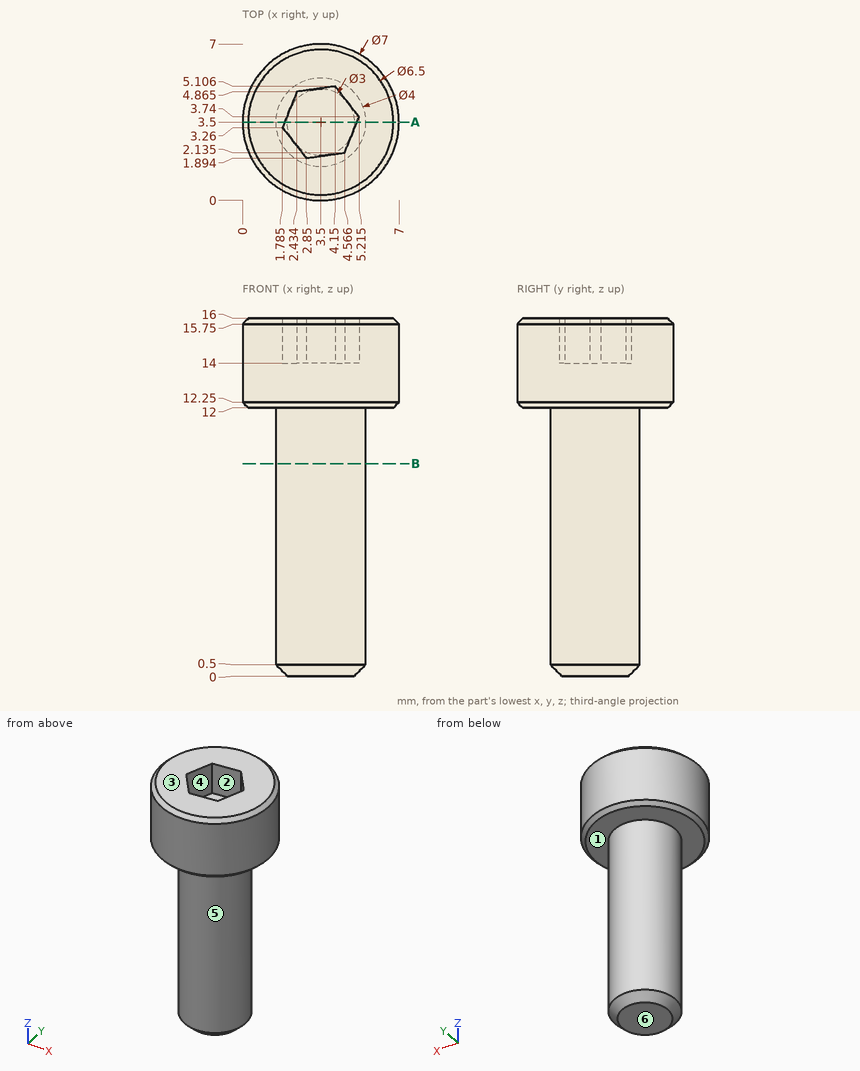
Can you work these out from the drawing? Everything is in mm from the part's minimum corner. A direction names the side the tool comes from. Round coordinates to 2 decimals unless told otherwise and drop trailing zeros. Order: outer loops, then holes, each group sorted by start corner. A loop starts at its lowest first (then second) coordinate and runs counter-clockwise, first axis right, second up. Notation, with made-up numbers: (-18, 50) -> (17, 50) arc R12 ccw to (17, 70) -> close; hole circle Ø4 at (6.25, 76). An arc over 180 degrees is marked (long way). Return JSON: item names as keys, results as strings. Group by question number.
1. If we section it at A-A, the plane y = 3.5: Write out the boundary of the cut face in (x, z).
2. I need wall thicknesses on line 1 (Z direction, x = 4, y = 3.75); line 2 (Z direction, x = 2, y = 6); line 3 (X direction, y = 4.25, z = 9.25) (1 decimal). Which ranges of each line are inside material? Lowest first, please. Write a range as [from, to].
3. If we section it at B-B, the plane z = 9.5: Write out the boundary of the cut face in (x, y).
4. We'd pull the mould along X, two halves only. Please class the marked faces 4, 5 and 6: released by +X, released by -X, zero draft, split by the parting line, or undercut.
5. Will these pins go through, and if not, where does the flat tip stop? pin 1 (1 mm diameter, centred on y = 2, z = 5.5, fed in from +X); pin 2 (3 mm diameter, centred on x = 6, z = 4.5, fed in from +Y); pin 3 (1 mm diameter, centred on y = 2.5, z = 5, fed in from -X).
6. Which directions (+Z, -Z, +X, -X, +Y, -Y) give clear straight access to the entire face, cutting with the end or side of a thin tool? Please do the marked faces 1, 2 and 3.
Output values:
{
 "1": {"outline": "(0, 12.25) -> (0.25, 12) -> (1.5, 12) -> (1.5, 0.5) -> (2, 0) -> (5, 0) -> (5.5, 0.5) -> (5.5, 12) -> (6.75, 12) -> (7, 12.25) -> (7, 15.75) -> (6.75, 16) -> (5.12, 16) -> (5.12, 14) -> (1.88, 14) -> (1.88, 16) -> (0.25, 16) -> (0, 15.75) -> close"},
 "2": {"line 1": "[0, 14]", "line 2": "[12, 16]", "line 3": "[1.6, 5.4]"},
 "3": {"outline": "circle Ø4 at (3.5, 3.5)"},
 "4": {"face 4": "undercut", "face 5": "split by the parting line", "face 6": "zero draft"},
 "5": {"pin 1": "x = 5.23", "pin 2": "y = 5.23", "pin 3": "x = 1.56"},
 "6": {"face 1": "-Z", "face 2": "+Z", "face 3": "+Z, +X, -X, +Y, -Y"}
}
